The model under review builds one solid part; all positions refer to its coordinate system, in mm. A direction names the side the tool comes from. Give positions to 0.01 mm unless a question says otherwise; leave off trailing zeros. Loops run counter-clockwise (first coordinate to the right, second up) from the corner with the lowest first, then second, coordinate; pieces in that order, holes last. Notation, with made-up numbers: M 16,-19.75 L 58,-19.75 A7 ccw 58,-15.75 Z; hole C -13,16.5 d10. An arc over 180 degrees is marked long. Put each result on its own line as item: value. Start each with the question number.
from build123d import *

# Parameters (mm, degrees)
SKETCH1_R           = 10
SKETCH1_R_2         = 8
BOSS_EXTRUDE1_DEPTH = 17


with BuildPart() as part:
    # Sketch1 → Boss-Extrude1 (new body)
    with BuildSketch(Plane.XY):
        Circle(SKETCH1_R)
        Circle(SKETCH1_R_2, mode=Mode.SUBTRACT)
    extrude(amount=BOSS_EXTRUDE1_DEPTH)

    # Sketch3 → Revolve1 (revolve)
    with BuildSketch(Plane(origin=(0, 0, 0), x_dir=(1, 0, 0), z_dir=(0, 1, 0))):
        Polygon((-10, -17), (-13, -17), (-13, -19), (-11, -19), (-8, -17), align=None)
    revolve(axis=Axis((0, 0, 0), (0, 0, 1)))

    # Sketch5 → Revolve2 (revolve)
    with BuildSketch(Plane(origin=(0, 0, 0), x_dir=(1, 0, 0), z_dir=(0, 1, 0)), mode=Mode.PRIVATE) as revolve2_sk:
        Polygon((-13, -19), (-42, -48), (-40, -48), (-11, -19), align=None)
    revolve(revolve2_sk.sketch.rotate(Axis((0, 0, 0), (0, 0, 1)), 180), axis=Axis((0, 0, 0), (0, 0, 1)))


solid = part.part
(1) We need section D-D, the plane z = 35. Write out the cut boundary in (x, y), plus the area to 3 significant figures.
(2) To check wall thickness, follow L1, parallel to Y at x = 0, z = 12; L2, parallel to X at y = -11.5, z = 39; L3, parallel to Y at x = 4.5, z = 25. State the ranges of each line that lie inside material, in increasing order. Write a range as [from, to].
(3) For faces 1 (the cylindrical face through (-2.17, -9.76, 8.38)), 2 (the cylindrical face through (-1.73, -7.81, 8.38)), list the 3-axis set-ups (+Z, -Z, +X, -X, +Y, -Y) from which the entire face can be reached by the end or side of a thin tool; tool diameter is ignored.
(4) Insertion check: pin 1 (10 mm diameter, centred on x = 1, y = -15, fed in from +Z); pin 2 (2 mm diameter, centred on x = 12.5, y = 27, fed in from -Z); pin 3 (10 mm diameter, centred on x = 11, y = 28, fed in from +Z). Each pin has a flat end and moves straight along its axis. Give the tip position at first contact, or say it passes through.
(5) Draft analysis for pull direction X (two halves, no side actions). For faces 3 (the flat face through (0, 8.2, 0)), 4 (the cylindrical face through (10.316, 7.91, 18.014)), 5 (the conical face through (5.73, -11.01, 20.41)), state which applies: +X half, -X half, draft (parallel to the pull), parting line (faces both ways), or undercut.
(6) We need section C-C, the plane z = 41. Write out the cut boundary in (x, y), plus the area to 3 significant figures.
(7) We need section A-A, the plane y = 0. Write out the cut boundary in (x, z).
Check sheet entries:
1. outline: C 0,0 d58; hole C 0,0 d54
1. area: 352 mm²
2. L1: y = [-10, -8], [8, 10]
2. L2: x = [-30.93, -28.79], [28.79, 30.93]
2. L3: y = [-18.46, -16.39], [16.39, 18.46]
3. face 1: -Z
3. face 2: +Z, -Z
4. pin 1: stops at z = 28.03
4. pin 2: stops at z = 34.75
4. pin 3: stops at z = 43.08
5. face 3: draft
5. face 4: parting line
5. face 5: undercut
6. outline: C 0,0 d70; hole C 0,0 d66
6. area: 427 mm²
7. outline: M -42,48 L -13,19 L -13,17 L -10,17 L -10,0 L -8,0 L -8,17 L -11,19 L -40,48 Z; M 8,0 L 10,0 L 10,17 L 13,17 L 13,19 L 42,48 L 40,48 L 11,19 L 8,17 Z
